```python
from build123d import *
from build123d.topology import SkipClean

# Parameters (mm, degrees)
SKETCH_1_R               = 18
SKETCH_1_R_2             = 10
EXTRUDE_1_DEPTH          = 5
CUT_EXTRUDE_1_DEPTH      = 35
CUT_EXTRUDE_1_DEPTH_BACK = 19
SKETCH_2_R               = 1.5
EXTRUDE_START            = 1
SKETCH_3_R               = 10.41594451
SKETCH_3_R_2             = 10
EXTRUDE_2_DEPTH          = 1
EXTRUDE_START_2          = 37.5
SKETCH_4_R               = 21
SKETCH_4_R_2             = 10
EXTRUDE_3_DEPTH          = 37.5
CHAMFER_1_SIZE           = 0.5
SKETCH_5_R               = 1
CUT_EXTRUDE_2_DEPTH      = 1


with BuildPart() as part:
    # 草图1 → 凸台-拉伸1 (new body)
    with BuildSketch(Plane.XY):
        Circle(SKETCH_1_R)
        Circle(SKETCH_1_R_2, mode=Mode.SUBTRACT)
    extrude(amount=EXTRUDE_1_DEPTH)

    # 草图2 → 切除-拉伸1 (cut, two sides: drawn at the far end of the back side and taken through both)
    with BuildSketch(Plane(origin=(0, 0, 0), x_dir=(0, 0, -1), z_dir=(1, 0, 0)).offset(-CUT_EXTRUDE_1_DEPTH_BACK)):
        with Locations(Location((-2.5, 0, 0), (0, 0, 180))):
            Circle(SKETCH_2_R)
    extrude(amount=CUT_EXTRUDE_1_DEPTH + CUT_EXTRUDE_1_DEPTH_BACK, mode=Mode.SUBTRACT)

    # 草图3 → 凸台-拉伸2 (add)
    with SkipClean():  # the faces are left unmerged after this step: merging them gives an invalid solid
        with BuildSketch(Plane(origin=(0, 0, 0), x_dir=(-1, 0, 0), z_dir=(0, 0, -1)).offset(EXTRUDE_START)):
            Circle(SKETCH_3_R)
            Circle(SKETCH_3_R_2, mode=Mode.SUBTRACT)
        extrude(amount=-EXTRUDE_2_DEPTH)

    # 草图4 → 凸台-拉伸3 (add)
    with SkipClean():  # the faces are left unmerged after this step: merging them gives an invalid solid
        with BuildSketch(Plane(origin=(0, 0, -1), x_dir=(-1, 0, 0), z_dir=(0, 0, -1)).offset(EXTRUDE_START_2)):
            Circle(SKETCH_4_R)
            Circle(SKETCH_4_R_2, mode=Mode.SUBTRACT)
        extrude(amount=-EXTRUDE_3_DEPTH)

    # 倒角1
    chamfer_1_edges = [part.edges().sort_by_distance(p)[0] for p in [
        (21, 0, -38.5),
        (21, 0, -1),
    ]]
    chamfer(chamfer_1_edges, length=CHAMFER_1_SIZE)

    # 草图5 → 切除-拉伸2 (cut)
    with BuildSketch(Plane(origin=(0, 0, -38.5), x_dir=(-1, 0, 0), z_dir=(0, 0, -1))):
        with Locations((3, -18)):
            Circle(SKETCH_5_R)
        with Locations((-3, -18)):
            Circle(SKETCH_5_R)
        with Locations((-3, 18)):
            Circle(SKETCH_5_R)
        with Locations((3, 18)):
            Circle(SKETCH_5_R)
    extrude(amount=-CUT_EXTRUDE_2_DEPTH, mode=Mode.SUBTRACT)


solid = part.part
```
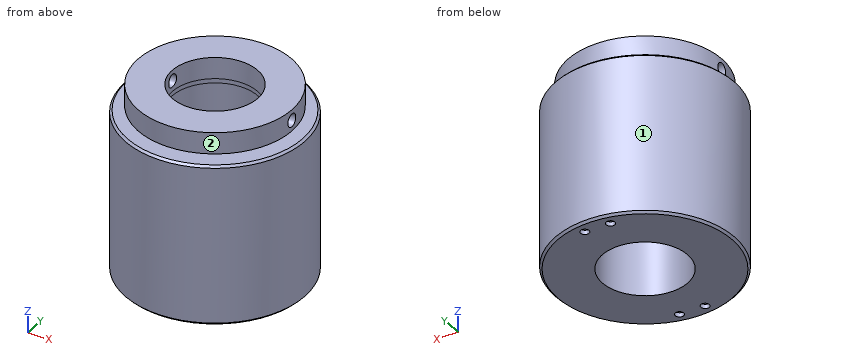
Verification items for the finished model (mm, model axes). Face numbers are marked on the shaded views. A direction names the side the tool comes from. Coordinates: 2 decimals unless noted, no trailing zeros. Loops run counter-clockwise (first coordinate to the right, second up) from the corner with the lowest first, then second, coordinate; pieces in that order, holes last. Notation, with made-up numbers: (-16.5, 18) - (1.5, 18) arc R33 cw to (1.5, 57) - close; hole circle Ø5 at (4.25, 4.25). An arc over 180 degrees is marked (long way). Put each result on its own line as item: value.
Item 1: Gauge pin test, flat ends, axial feed: pin 1 Ø1.6 at (x, y) = (-3, -18) entering from -Z; pin 2 Ø5 at (x, z) = (5.5, -9.5) entering from -Y; pin 3 Ø12 at (x, z) = (-4, -11) entering from -Y. Record the tip position at first contact, or that the pin passes through.
Conclusion:
pin 1: stops at z = -37.5
pin 2: stops at y = -20.78
pin 3: stops at y = -21
Item 2: Section check A-A (x = 0). Enter the section's corners in (y, z).
Conclusion:
outline: (-21, -38) - (-20.5, -38.5) - (-10, -38.5) - (-10, 5) - (-18, 5) - (-18, 0) - (-10.42, 0) - (-10.42, -1) - (-20.5, -1) - (-21, -1.5) - close; (10, -38.5) - (20.5, -38.5) - (21, -38) - (21, -1.5) - (20.5, -1) - (10.42, -1) - (10.42, 0) - (18, 0) - (18, 5) - (10, 5) - close
Item 3: Section check B-B (z = -9). Enter the section's corners in (x, y).
Conclusion:
outline: circle Ø42 at (0, 0); hole circle Ø20 at (0, 0)
Item 4: Scan lines: line 1 along Z through (x, y) = (13, -9.5); line 2 along Y through (x, z) = (0, 2.4); line 3 along Y through (x, z) = (0, -0.25). Record each from-to range of solid material in increasing order.
Conclusion:
line 1: z = -38.5 to -1, 0 to 5
line 2: y = -18 to -10, 10 to 18
line 3: y = -10.42 to -10, 10 to 10.42
Item 5: Set-up check for the marked faces 1 and 2: record each of +Z, -Z, +X, -X, +Y, -Y from which the full face is reachable in a straight line by a thin tool's end or side.
Conclusion:
face 1: +Z, -Z
face 2: +Z
Item 6: Section check C-C (x = -11.5). Give the number of separate pieces and of enclosed holes in the cut face, then the cut area to 3 significant figures.
Conclusion:
separate pieces: 2
enclosed holes: 1
area: 1,450 mm2
